from build123d import *

# Parameters (mm, degrees)
BOX007_W                = 46
BOX007_H                = 60
BOX007_DEPTH            = 22
PAD010_DEPTH            = 46
POCKET_DEPTH            = 22
POCKET001_DEPTH         = 22
CYLINDER_R              = 2
CYLINDER_DEPTH          = 4
POCKET002_DEPTH         = 2
FILLET002_R             = 0.2
FILLET003_R             = 0.4
BODY010_PLACEMENT_ANGLE = 90


with BuildPart() as part:
    # Box007 → Box007 (join)
    with BuildSketch(Plane.XY):
        with Locations((23, 30)):
            Rectangle(BOX007_W, BOX007_H)
    extrude(amount=BOX007_DEPTH)

    # Sketch012 → Pad010 (join)
    with BuildSketch(Plane.YZ):
        Polygon((0, 1.5), (-1.5, 1.5), (-1.5, -1.5), (61.5, -1.5), (61.5, 1.5), (60, 1.5), (60, 0), (0, 0), align=None)
    extrude(amount=PAD010_DEPTH)

    # Sketch013 → Pocket (cut)
    with BuildSketch(Plane.XY):
        with BuildLine():
            ThreePointArc((28, 6), (23, 11), (18, 6))
            Line((18, 6), (18, -1))
            Line((18, -1), (28, -1))
            Line((28, -1), (28, 6))
        make_face()
    extrude(amount=POCKET_DEPTH, mode=Mode.SUBTRACT)

    # Sketch014 → Pocket001 (cut)
    with BuildSketch(Plane.XY):
        with BuildLine():
            ThreePointArc((18, 53), (23, 48), (28, 53))
            Line((28, 53), (28, 61))
            Line((28, 61), (18, 61))
            Line((18, 61), (18, 53))
        make_face()
    extrude(amount=POCKET001_DEPTH, mode=Mode.SUBTRACT)

    # Cylinder → Cylinder (cut)
    with BuildSketch(Plane(origin=(23, 6, -2), x_dir=(1, 0, 0), z_dir=(0, 0, 1))):
        Circle(CYLINDER_R)
    extrude(amount=CYLINDER_DEPTH, mode=Mode.SUBTRACT)

    # Sketch015 → Pocket002 (cut, symmetric)
    with BuildSketch(Plane.XY):
        with BuildLine():
            ThreePointArc((25, 56), (23, 58), (21, 56))
            Line((21, 56), (21, 53))
            ThreePointArc((21, 53), (23, 51), (25, 53))
            Line((25, 53), (25, 56))
        make_face()
    extrude(amount=POCKET002_DEPTH, both=True, mode=Mode.SUBTRACT)

    # Fillet002
    fillet002_edges = [part.edges().sort_by_distance(p)[0] for p in [
        (23, -1.5, 1.5),
        (23, 61.5, 1.5),
    ]]
    fillet(fillet002_edges, radius=FILLET002_R)

    # Fillet003
    fillet003_edges = [part.edges().sort_by_distance(p)[0] for p in [
        (9, 0, 22),
        (37, 0, 22),
        (46, 30, 22),
        (37, 60, 22),
        (9, 60, 22),
        (0, 30, 22),
    ]]
    fillet(fillet003_edges, radius=FILLET003_R)


with BuildPart() as part_1:
    # Body010 placement: moved
    add(part.part.moved(Location((30, -42, -74.8))).rotate(Axis((30, -42, -74.8), (0, 0, 1)), BODY010_PLACEMENT_ANGLE))


solid = part_1.part
For this review, take the finished solid that the model builds, in its own axes (mm). A direction names the side the tool comes from. Round coordinates to 2 decimals unless told otherwise and drop trailing zeros. Order: outer loops, then holes, each group sorted by start corner. A loop starts at its lowest first (then second) coordinate and runs counter-clockwise, first axis right, second up. Notation, with made-up numbers: M -11,-31 L -3,-31 A21 cw -3,5 Z; hole C 49.25,77 d10. An arc over 180 degrees is marked long. Write each question's results on one line, items separated by ' | '. Start each with the question number.
1. Add section B-B (z = -70). State the section outline as (x, y) points, then the cut area to 3 significant figures.
2. Draft analysis for pull direction Y (two halves, no side actions). For faces 1 (the face through (0, 4, -65)), 2 (the face through (-30.7, -24.4, -73.3)), 3 (the face through (-31, -19, -74)), 4 (the face through (-24, -17, -76)), state which applies: pulls with the +Y half, pulls with the -Y half, needs draft (parallel to the pull), parting line crosses it, or undercut.
3. Add section C-C (y = -7). State the section outline as (x, z) points, then the cut area to 3 significant figures.
4. Add section A-A (y = -19). State the section outline as (x, z) points, then the cut area to 3 significant figures.
5. To check wall thickness, follow L1, parallel to X at y = -19, z = -75.15; L2, parallel to Y at x = -23, z = -55.75; L3, parallel to X at y = -2.5, z = -64.5. State the ranges of each line that lie inside material, in increasing order. Write a range as [from, to].
6. Tool access review of faces 5 (the face through (30.6, -24.4, -73.3)), 6 (the face through (-28, -19, -76)), 7 (the face through (27, -24, -64)): name each direction out of +Z, -Z, +X, -X, +Y, -Y from which nothing blocks a thin tool from reaching the whole face with its end or side.
7. Clearance check with flat-ended pins moving along their axes: pin 1 Ø5.5 at (y, z) = (-7, -61.5) entering from -X; pin 2 Ø5.5 at (y, z) = (-5.5, -66.5) entering from +X; pin 3 Ø0.7 at (x, y) = (30.5, -19) entering from +Z. State where each tip first meets the part, or that it passes through.
Output values:
1) outline: M -30,-42 L 30,-42 L 30,-24 L 24,-24 A5 cw 24,-14 L 30,-14 L 30,4 L -30,4 L -30,-14 L -23,-14 A5 cw -23,-24 L -30,-24 Z | area: 2,550 mm^2
2) face 1: pulls with the +Y half | face 2: needs draft | face 3: undercut | face 4: undercut
3) outline: M -31.5,-76.3 L 31.5,-76.3 L 31.5,-73.5 A0.2 ccw 31.3,-73.3 L 30,-73.3 L 30,-53.2 A0.4 ccw 29.6,-52.8 L -29.6,-52.8 A0.4 ccw -30,-53.2 L -30,-73.3 L -31.3,-73.3 A0.2 ccw -31.5,-73.5 Z | area: 1,420 mm^2
4) outline: M -31.5,-76.3 L -28,-76.3 L -28,-74.8 L -31,-74.8 L -31,-73.3 L -31.3,-73.3 A0.2 ccw -31.5,-73.5 Z; M -21,-76.3 L 22,-76.3 L 22,-74.8 L 19,-74.8 L 19,-52.8 L -18,-52.8 L -18,-74.8 L -21,-74.8 Z; M 26,-76.3 L 31.5,-76.3 L 31.5,-73.5 A0.2 ccw 31.3,-73.3 L 31,-73.3 L 31,-74.8 L 26,-74.8 Z | area: 893 mm^2
5) L1: [-31.5, -28], [-21, 22], [26, 31.5] | L2: [-42, -24], [-14, 4] | L3: [-30, 30]
6) face 5: +Z, +X, +Y, -Y | face 6: +Z, -Z | face 7: +Z
7) pin 1: x = -30 | pin 2: x = 30 | pin 3: z = -74.8
